Input: part model. Units: mm. Frame: model coordinates. Coordinates: 2 decimals unless noted, no trailing zeros. Loops run counter-clockwise (first coordinate to the right, second up) from the corner with the lowest first, then second, coordinate; pieces in that order, holes last. Notation, with made-up numbers: (57, -23.5) - (104, -23.5) arc R20 ccw to (104, -3.5) - close; hole circle Ø7 at (-18.5, 16.25). An arc over 180 degrees is marked (long way). Write item = value, one per line. Start each with the question number.
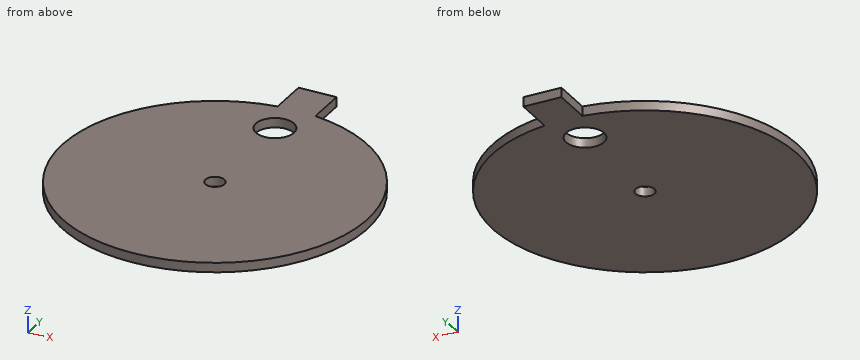
from build123d import *

# Parameters (mm, degrees)
F0_R     = 50.8
F1_DEPTH = 3.175
F2_R     = 6.35
F3_DEPTH = 3.175
F4_R     = 3.175
F5_DEPTH = 25.4
F7_DEPTH = 3.175


with BuildPart() as f1:
    # F0 (on Top) → F1 (new body)
    with BuildSketch(Plane.XY):
        Circle(F0_R)
    extrude(amount=F1_DEPTH)

    # F2 (on face) → F3 (cut)
    with BuildSketch(Plane.XY.offset(3.175)):
        with Locations((0, 38.1)):
            Circle(F2_R)
    extrude(amount=-F3_DEPTH, mode=Mode.SUBTRACT)

    # F4 (on face) → F5 (cut)
    with BuildSketch(Plane.XY.offset(3.175)):
        Circle(F4_R)
    extrude(amount=-F5_DEPTH, mode=Mode.SUBTRACT)

    # F6 (on face) → F7 (join)
    with BuildSketch(Plane.XY.offset(3.175)):
        with BuildLine():
            Line((-5.628267, 63.773812), (-5.628267, 50.487252))
            ThreePointArc((-5.628267, 50.487252), (0.72744, 50.794791), (7.071733, 50.305373))
            Line((7.071733, 50.305373), (7.071733, 63.773812))
            Line((7.071733, 63.773812), (-5.628267, 63.773812))
        make_face()
    extrude(amount=-F7_DEPTH)


solid = f1.part
Item 1: Cut plane B-B on z = 1.2. Return loops of the section in (x, y) (3 decimals).
Item 2: Cut plane A-A on x = 0. Return loops of the section in (y, z) (3 decimals).
Item 3: Cut plane C-C on y = 38.1. Return loops of the section in (x, z) (3 decimals), plus the area to 3 significant figures.
Item 4: Pin query (flat end, axial travel): pin 1 (1.5 mm diameter, centred on x = -18, z = 2, fed in from +Y); pin 2 (10 mm diameter, centred on x = 0, y = 38.1, fed in from -Z); pin 3 (1.5 mm diameter, centred on x = 31.5, z = 1, fed in from -Y); pin 4 (1 mm diameter, centred on y = 14, z = 2, fed in from +X). Return the tip coordinate at first contact, or that it passes through.
Item 5: Ray query, line 1 (Y direction, x = 0, z = 1.6) (3 decimals); line 2 (X direction, y = -9.5, z = 2.35); line 3 (Y direction, x = -11, z = 1.6). Return the intervals inside material, ascending.
Item 6: Cut plane D-D on y = 53. Return loops of the section in (x, z) (3 decimals), plus the area to 3 significant figures.
Recorded:
q1.outline = (-5.628, 50.487) arc R50.8 ccw (long way) to (7.072, 50.305) - (7.072, 63.774) - (-5.628, 63.774) - close; hole circle Ø12.7 at (0, 38.1); hole circle Ø6.35 at (0, 0)
q2.outline = (-50.8, 0) - (-3.175, 0) - (-3.175, 3.175) - (-50.8, 3.175) - close; (3.175, 0) - (31.75, 0) - (31.75, 3.175) - (3.175, 3.175) - close; (44.45, 0) - (63.774, 0) - (63.774, 3.175) - (44.45, 3.175) - close
q3.outline = (-33.601, 0) - (-6.35, 0) - (-6.35, 3.175) - (-33.601, 3.175) - close; (6.35, 0) - (33.601, 0) - (33.601, 3.175) - (6.35, 3.175) - close
q3.area = 173 mm²
q4.pin_1 = 47.78
q4.pin_2 = through
q4.pin_3 = -40.44
q4.pin_4 = 48.97
q5.line_1 = -50.8 to -3.175, 3.175 to 31.75, 44.45 to 63.774
q5.line_2 = -49.9 to 49.9
q5.line_3 = -49.59 to 49.59
q6.outline = (-5.628, 0) - (7.072, 0) - (7.072, 3.175) - (-5.628, 3.175) - close
q6.area = 40.3 mm²
